Verification items for the finished model (mm, model axes). A direction names the side the tool comes from. Round coordinates to 2 decimals unless told otherwise and drop trailing zeros. Order: outer loops, then holes, each group sorted by start corner. A loop starts at its lowest first (then second) coordinate and runs counter-clockwise, first axis right, second up. Notation, with made-up numbers: (8, 62.5) -> (28, 62.5) arc R19 cw to (28, 82.5) -> close; hole circle Ø1 at (-19.75, 13.25). An arc over 180 degrees is marked (long way). Write item = value, one per line. Start each with the question number.
from build123d import *

# Parameters (mm, degrees)
BOSS_EXTRUDE1_DEPTH     = 18
SKETCH2_R               = 9.5
SKETCH2_W               = 9
SKETCH2_H               = 5.5
CUT_EXTRUDE1_DEPTH      = 51.410812332
FILLET1_R               = 5
FILLET2_R               = 0.5
FILLET3_R               = 2
FILLET4_R               = 2.75
CUT_EXTRUDE2_DEPTH      = 15
SKETCH7_R               = 1.6
CUT_EXTRUDE3_DEPTH      = 10
SKETCH8_R               = 2.35
CUT_EXTRUDE4_DEPTH      = 5
SKETCH9_R               = 2.5
CUT_EXTRUDE5_DEPTH      = 0.5
MIRROR3_COPY_1_SKETCH_R = 1.6
MIRROR3_COPY_1_DEPTH    = 10
MIRROR3_COPY_2_SKETCH_R = 2.35
MIRROR3_COPY_2_DEPTH    = 5
MIRROR3_COPY_3_SKETCH_R = 2.5
MIRROR3_COPY_3_DEPTH    = 0.5
BOSS_EXTRUDE2_DEPTH     = 27
SKETCH11_W              = 11
SKETCH11_H              = 20
CUT_EXTRUDE6_DEPTH      = 21.2
SKETCH12_W              = 11
SKETCH12_H              = 3.7
CUT_EXTRUDE7_DEPTH      = 12.5
FILLET5_R               = 10
CUT_EXTRUDE8_REACH      = 67.133
SKETCH13_W              = 11
SKETCH13_H              = 19.8
FILLET6_R               = 10
SKETCH14_W              = 11
SKETCH14_H              = 7.4
CUT_EXTRUDE9_DEPTH      = 12.5
SKETCH15_R              = 2.75
BOSS_EXTRUDE3_DEPTH     = 0.8
BOSS_EXTRUDE3_TAPER     = 30
SKETCH16_W              = 14
SKETCH16_H              = 6.815
CUT_EXTRUDE10_DEPTH     = 0.8
SKETCH19_R              = 2.75
BOSS_EXTRUDE4_DEPTH     = 0.8
BOSS_EXTRUDE4_TAPER     = 30
FILLET7_R               = 2


with BuildPart() as part:
    # Sketch1 → Boss-Extrude1 (new body)
    with BuildSketch(Plane.XY):
        with BuildLine():
            Line((-17.5, 17.5), (-31.5, 3.5))
            Line((-31.5, 3.5), (-31.5, -3.5))
            Line((-31.5, -3.5), (-17.5, -17.5))
            Line((-17.5, -17.5), (17.5, -17.5))
            Line((17.5, -17.5), (31.5, -3.5))
            Line((31.5, -3.5), (31.5, 3.5))
            Line((31.5, 3.5), (17.5, 17.5))
            Line((17.5, 17.5), (13.560660172, 17.5))
            Line((13.560660172, 17.5), (17.25, 13.810660172))
            Line((17.25, 13.810660172), (17.25, 9.845660172))
            Line((17.25, 9.845660172), (22.916347453, 4.179312718))
            ThreePointArc((22.916347453, 4.179312718), (22.602164744, -4.198757241), (21.880882362, 4.154117638))
            Line((21.880882362, 4.154117638), (16.5, 9.535))
            Line((16.5, 9.535), (16.5, 13.5))
            Line((16.5, 13.5), (12.5, 17.5))
            Line((12.5, 17.5), (-12.5, 17.5))
            Line((-12.5, 17.5), (-16.5, 13.5))
            Line((-16.5, 13.5), (-16.5, 9.535))
            Line((-16.5, 9.535), (-21.880882362, 4.154117638))
            ThreePointArc((-21.880882362, 4.154117638), (-22.602164744, -4.198757241), (-22.916347453, 4.179312718))
            Line((-22.916347453, 4.179312718), (-17.25, 9.845660172))
            Line((-17.25, 9.845660172), (-17.25, 13.810660172))
            Line((-17.25, 13.810660172), (-13.560660172, 17.5))
            Line((-13.560660172, 17.5), (-17.5, 17.5))
        make_face()
    extrude(amount=BOSS_EXTRUDE1_DEPTH)

    # Sketch2 → Cut-Extrude1 (cut, through all)
    with BuildSketch(Plane(origin=(0, 17.5, 0), x_dir=(1, 0, 0), z_dir=(0, 1, 0))):
        Circle(SKETCH2_R)
        with Locations((-5.5, -15.25)):
            Rectangle(SKETCH2_W, SKETCH2_H)
    extrude(amount=-CUT_EXTRUDE1_DEPTH, mode=Mode.SUBTRACT)

    # Fillet1
    fillet1_edges = [part.edges().sort_by_distance(p)[0] for p in [
        (17.5, 17.5, 9),
        (31.5, 3.5, 9),
        (31.5, -3.5, 9),
        (17.5, -17.5, 9),
        (-17.5, -17.5, 9),
        (-31.5, -3.5, 9),
        (-31.5, 3.5, 9),
        (-17.5, 17.5, 9),
    ]]
    fillet(fillet1_edges, radius=FILLET1_R)

    # Fillet2
    fillet2_edges = [part.edges().sort_by_distance(p)[0] for p in [
        (-13.560660172, 17.5, 9),
        (-22.916347453, 4.179312718, 9),
        (-21.880882362, 4.154117638, 9),
        (21.880882362, 4.154117638, 9),
        (22.916347453, 4.179312718, 9),
        (13.560660172, 17.5, 9),
    ]]
    fillet(fillet2_edges, radius=FILLET2_R)

    # Fillet3
    fillet3_edges = [part.edges().sort_by_distance(p)[0] for p in [
        (-17.25, 9.845660172, 9),
        (17.25, 9.845660172, 9),
    ]]
    fillet(fillet3_edges, radius=FILLET3_R)

    # Fillet4
    fillet4_edges = [part.edges().sort_by_distance(p)[0] for p in [
        (-16.5, 9.535, 9),
        (16.5, 9.535, 9),
    ]]
    fillet(fillet4_edges, radius=FILLET4_R)

    # Sketch4 → Cut-Revolve1 (revolve, cut)
    with BuildSketch(Plane(origin=(0, 0, 6), x_dir=(-1, 0, 0), z_dir=(0, 0, -1))):
        Polygon((23.439696962, 11.560303038), (25.561017306, 9.438982694), (23.439696962, 7.317662351), (22.555813485, 8.201545827), (14.070532111, -0.283735547), (12.833095244, 0.95370132), align=None)
    cut_revolve1 = revolve(axis=Axis((-23.439696962, 11.560303038, 6), (0.7071067811865471, -0.707106781186548, 0)), mode=Mode.SUBTRACT)

    # Sketch6 → Cut-Extrude2 (cut)
    with BuildSketch(Plane(origin=(-6.893398282, 6.893398282, 0), x_dir=(0, 0, 1), z_dir=(-0.7071067811865471, 0.707106781186548, 0))):
        Polygon((3.425, -9.886676943), (6, -11.373353886), (8.575, -9.886676943), (8.575, -6.913323057), (6, -5.426646114), (3.425, -6.913323057), align=None)
    cut_extrude2 = extrude(amount=-CUT_EXTRUDE2_DEPTH, mode=Mode.SUBTRACT)

    # Mirror1: Cut-Revolve1, Cut-Extrude2 across plane
    add(cut_revolve1.mirror(Plane(origin=(0, 0, 0), x_dir=(0, 0, 1), z_dir=(1, 0, 0))), mode=Mode.SUBTRACT)
    add(cut_extrude2.mirror(Plane(origin=(0, 0, 0), x_dir=(0, 0, 1), z_dir=(1, 0, 0))), mode=Mode.SUBTRACT)

    # Sketch7 → Cut-Extrude3 (cut)
    with BuildSketch(Plane(origin=(0, 0, 0), x_dir=(-1, 0, 0), z_dir=(0, 0, -1))):
        with Locations((-12.5, 12.5)):
            Circle(SKETCH7_R)
    cut_extrude3 = extrude(amount=-CUT_EXTRUDE3_DEPTH, mode=Mode.SUBTRACT)

    # Sketch8 → Cut-Extrude4 (cut)
    with BuildSketch(Plane(origin=(0, 0, 0), x_dir=(-1, 0, 0), z_dir=(0, 0, -1))):
        with Locations((-12.5, 12.5)):
            Circle(SKETCH8_R)
    cut_extrude4 = extrude(amount=-CUT_EXTRUDE4_DEPTH, mode=Mode.SUBTRACT)

    # Sketch9 → Cut-Extrude5 (cut)
    with BuildSketch(Plane(origin=(0, 0, 0), x_dir=(-1, 0, 0), z_dir=(0, 0, -1))):
        with Locations((-12.5, 12.5)):
            Circle(SKETCH9_R)
    cut_extrude5 = extrude(amount=-CUT_EXTRUDE5_DEPTH, mode=Mode.SUBTRACT)

    # Mirror2: Cut-Extrude3, Cut-Extrude4, Cut-Extrude5 across plane
    add(cut_extrude3.mirror(Plane.ZX), mode=Mode.SUBTRACT)
    add(cut_extrude4.mirror(Plane.ZX), mode=Mode.SUBTRACT)
    add(cut_extrude5.mirror(Plane.ZX), mode=Mode.SUBTRACT)

    # Mirror3: Cut-Extrude3, Cut-Extrude4, Cut-Extrude5 across plane
    add(cut_extrude3.mirror(Plane(origin=(0, 0, 0), x_dir=(0, 0, 1), z_dir=(1, 0, 0))), mode=Mode.SUBTRACT)
    add(cut_extrude4.mirror(Plane(origin=(0, 0, 0), x_dir=(0, 0, 1), z_dir=(1, 0, 0))), mode=Mode.SUBTRACT)
    add(cut_extrude5.mirror(Plane(origin=(0, 0, 0), x_dir=(0, 0, 1), z_dir=(1, 0, 0))), mode=Mode.SUBTRACT)

    # Mirror3 copy 1 sketch → Mirror3 copy 1 (cut)
    with BuildSketch(Plane(origin=(0, 0, 0), x_dir=(1, 0, 0), z_dir=(0, 0, -1))):
        with Locations((-12.5, 12.5)):
            Circle(MIRROR3_COPY_1_SKETCH_R)
    extrude(amount=-MIRROR3_COPY_1_DEPTH, mode=Mode.SUBTRACT)

    # Mirror3 copy 2 sketch → Mirror3 copy 2 (cut)
    with BuildSketch(Plane(origin=(0, 0, 0), x_dir=(1, 0, 0), z_dir=(0, 0, -1))):
        with Locations((-12.5, 12.5)):
            Circle(MIRROR3_COPY_2_SKETCH_R)
    extrude(amount=-MIRROR3_COPY_2_DEPTH, mode=Mode.SUBTRACT)

    # Mirror3 copy 3 sketch → Mirror3 copy 3 (cut)
    with BuildSketch(Plane(origin=(0, 0, 0), x_dir=(1, 0, 0), z_dir=(0, 0, -1))):
        with Locations((-12.5, 12.5)):
            Circle(MIRROR3_COPY_3_SKETCH_R)
    extrude(amount=-MIRROR3_COPY_3_DEPTH, mode=Mode.SUBTRACT)

    # Sketch10 → Boss-Extrude2 (add)
    with BuildSketch(Plane.XY.offset(18)):
        Polygon((12.5, 17.5), (-12.5, 17.5), (-16.5, 13.5), (-16.5, -13.5), (-12.5, -17.5), (12.5, -17.5), (16.5, -13.5), (16.5, 13.5), align=None)
    extrude(amount=BOSS_EXTRUDE2_DEPTH)

    # Sketch11 → Cut-Extrude6 (cut)
    with BuildSketch(Plane(origin=(0, 17.5, 0), x_dir=(1, 0, 0), z_dir=(0, 1, 0))):
        with Locations((5.5, -22.5)):
            Rectangle(SKETCH11_W, SKETCH11_H)
    extrude(amount=-CUT_EXTRUDE6_DEPTH, mode=Mode.SUBTRACT)

    # Sketch12 → Cut-Extrude7 (cut)
    with BuildSketch(Plane(origin=(0, 0, 32.5), x_dir=(-1, 0, 0), z_dir=(0, 0, -1))):
        with Locations((-5.5, 1.85)):
            Rectangle(SKETCH12_W, SKETCH12_H)
        Polygon((-11, -3.7), (0, -3.7), (0, -3.591245546), (0, 0), (-11, 0), align=None)
    extrude(amount=-CUT_EXTRUDE7_DEPTH, mode=Mode.SUBTRACT)

    # Fillet5
    fillet5_edges = [part.edges().sort_by_distance(p)[0] for p in [
        (5.5, -3.7, 12.5),
    ]]
    fillet(fillet5_edges, radius=FILLET5_R)

    # Cut-Extrude8: up to this face of the body (flat: up to its plane)
    cut_extrude8_end = Plane(part.part.faces().sort_by_distance((5.5, 3.7, 38.75))[0])
    # Sketch13 → Cut-Extrude8 (cut, up to the picked face)
    with BuildSketch(Plane.XZ.offset(17.5), mode=Mode.PRIVATE) as cut_extrude8_sk1:
        with Locations((-5.5, 35.1)):
            Rectangle(SKETCH13_W, SKETCH13_H)
    cut_extrude8_tool1 = split(extrude(cut_extrude8_sk1.sketch, amount=-CUT_EXTRUDE8_REACH, mode=Mode.PRIVATE), bisect_by=cut_extrude8_end, keep=Keep.BOTH, mode=Mode.PRIVATE)
    add(cut_extrude8_tool1.solids().sort_by(Axis((-5.5, -17.5, 35.1), (0, 1, 0)))[0], mode=Mode.SUBTRACT)

    # Fillet6
    # the kernel refuses this fillet: 10 mm, written as the material it adds along each edge
    with BuildSketch(Plane(origin=(25, 3.7, 25.2), x_dir=(0, 0, 1), z_dir=(-1, 0, 0))) as fillet6_piece_1_section:
        with BuildLine():
            CenterArc((FILLET6_R, -FILLET6_R), FILLET6_R, 90, 90)
            Line((0, -FILLET6_R), (0, 0))
            Line((0, 0), (FILLET6_R, 0))
        make_face()
    fillet6_piece_1 = extrude(amount=36, mode=Mode.PRIVATE)
    fillet6_piece_1 = split(fillet6_piece_1, bisect_by=Plane(origin=(5.5, 3.588944861, 32.5), z_dir=(0, 0, 1)), keep=Keep.TOP, mode=Mode.PRIVATE)
    fillet6_piece_1 = split(fillet6_piece_1, bisect_by=Plane(origin=(11, 3.588944861, 33.172467691), z_dir=(-1, 0, 0)), keep=Keep.TOP, mode=Mode.PRIVATE)
    add(fillet6_piece_1)
    with BuildSketch(Plane(origin=(0, 3.7, 25.2), x_dir=(0, 0, 1), z_dir=(-1, 0, 0))) as fillet6_piece_2:
        with BuildLine():
            CenterArc((FILLET6_R, -FILLET6_R), FILLET6_R, 90, 90)
            Line((0, -FILLET6_R), (0, 0))
            Line((0, 0), (FILLET6_R, 0))
        make_face()
    extrude(amount=11)

    # Sketch14 → Cut-Extrude9 (cut)
    with BuildSketch(Plane.XY.offset(45)):
        with Locations((5.5, 0)):
            Rectangle(SKETCH14_W, SKETCH14_H)
    extrude(amount=-CUT_EXTRUDE9_DEPTH, mode=Mode.SUBTRACT)

    # Sketch15 → Boss-Extrude3 (add)
    with BuildSketch(Plane(origin=(-11, 0, 0), x_dir=(0, 0, -1), z_dir=(1, 0, 0))):
        with Locations((-35.23, -6.365)):
            Circle(SKETCH15_R)
    extrude(amount=BOSS_EXTRUDE3_DEPTH, taper=BOSS_EXTRUDE3_TAPER)

    # Sketch16 → Cut-Extrude10 (cut)
    with BuildSketch(Plane.ZY):
        with Locations((38, -7.1075)):
            Rectangle(SKETCH16_W, SKETCH16_H)
    extrude(amount=-CUT_EXTRUDE10_DEPTH, mode=Mode.SUBTRACT)

    # Sketch17 → Cut-Revolve2 (revolve, cut)
    with BuildSketch(Plane.XY.offset(35.23)):
        Polygon((-16.5, -6.365), (-16.5, -3.265), (-13.5, -3.265), (-13.5, -4.865), (11.5, -4.865), (11.5, -4.115), (16, -4.115), (16, -3.865), (16.5, -3.865), (16.5, -6.365), align=None)
    revolve(axis=Axis((31.947720378, -6.365, 35.23), (-1, 0, 0)), mode=Mode.SUBTRACT)

    # Sketch19 → Boss-Extrude4 (add)
    with BuildSketch(Plane.ZY.offset(-11)):
        with Locations((22.5, 6.365)):
            Circle(SKETCH19_R)
    boss_extrude4 = extrude(amount=BOSS_EXTRUDE4_DEPTH, taper=BOSS_EXTRUDE4_TAPER)

    # Mirror4: Boss-Extrude4 across plane
    add(boss_extrude4.mirror(Plane(origin=(5.5, 0, 0), x_dir=(0, 0, 1), z_dir=(1, 0, 0))))

    # Sketch20 → Cut-Revolve3 (revolve, cut)
    with BuildSketch(Plane.XY.offset(22.5), mode=Mode.PRIVATE) as cut_revolve3_sk:
        Polygon((16.5, 6.365), (16.5, 9.465), (13.5, 9.465), (13.5, 7.865), (-11.5, 7.865), (-11.5, 8.615), (-16, 8.615), (-16, 8.865), (-16.5, 8.865), (-16.5, 6.365), align=None)
    revolve(cut_revolve3_sk.sketch.rotate(Axis((11, 6.365, 22.5), (-1, 0, 0)), 90), axis=Axis((11, 6.365, 22.5), (-1, 0, 0)), mode=Mode.SUBTRACT)

    # Fillet7
    fillet7_edges = [part.edges().sort_by_distance(p)[0] for p in [
        (16.5, -13.5, 31.5),
        (12.5, -17.5, 31.5),
        (-12.5, -17.5, 31.5),
        (-16.5, -13.5, 31.5),
        (-16.5, 13.5, 22.5),
        (-12.5, 17.5, 22.5),
        (12.5, 17.5, 22.5),
        (16.5, 13.5, 22.5),
    ]]
    fillet(fillet7_edges, radius=FILLET7_R)


solid = part.part
(1) Scan lines: line 1 along X through (y, z) = (-12.5, 3.15); line 2 along X through (y, z) = (-1, 42); line 3 along X through (y, z) = (6, 19.5). Record each from-to range of solid material in increasing order. Write a range as from..to.
(2) Draft check along Y on faces 6 (the flat face through (5, 12, 12.5)), 7 (the cylindrical face through (16.35, -13.43, 31.69)), 8 (the flat face through (-11, -1, 3.425)), 9 (the cylindrical face through (-22.77, -4.19, 8.87)). Enter one of: +Y half, -Y half, draft (parallel to the pull), parting line (faces both ways), or undercut.
(3) Depth check by flat-ended pin: pin 1 (2.5 mm diameter, centred on y = 6.365, z = 22.5, fed in from -X); pin 2 (6.5 mm diameter, centred on y = -6.365, z = 35.23, fed in from +X); pin 3 (4 mm diameter, centred on x = 15.5, z = 38.5, fed in from +Y); pin 4 (2.5 mm diameter, centred on x = -4.5, y = 7.5, fed in from -Z). Enter the tip coordinate at first touch or a pass-through.
(4) Set-up check for faces 1 (the cylindrical face through (-5.4, 6.3, 24)), 2 (the cylindrical face through (14.1, -12.57, 7.46)), 3 (the flat face through (-9.59, 0.88, 4.73)), 4 (the flat face through (-11.5, 8, 23)), 5 (the cylindrical face through (16.715, 9.608, 9.126)): record each of +Z, -Z, +X, -X, +Y, -Y from which the full face is reachable in a straight line by a thin tool's end or side.
(5) Cross-section at A-A (z = 40.5). Enter the section's corners in (x, y) (3 decimals), and give its area (3 significant figures).
Outcome:
q1.line_1 = -22.5..-14.85, -10.15..-8.96, 8.96..10.15, 14.85..22.5
q1.line_2 = -16.5..-11, 11..16.5
q1.line_3 = -16.5..0, 11..13.5
q2.face_6 = draft
q2.face_7 = -Y half
q2.face_8 = undercut
q2.face_9 = undercut
q3.pin_1 = through
q3.pin_2 = 16.5
q3.pin_3 = 16.5
q3.pin_4 = 7.56
q4.face_1 = +X, -X
q4.face_2 = -Z
q4.face_3 = none
q4.face_4 = -X
q4.face_5 = +Z, -Z
q5.outline = (-16.5, -12.672) arc R2 ccw to (-15.914, -14.086) -> (-13.086, -16.914) arc R2 ccw to (-11.672, -17.5) -> (-11, -17.5) -> (-11, 3.7) -> (11, 3.7) -> (11, -3.7) -> (0.8, -3.7) -> (0.8, -10.515) -> (0, -10.515) -> (0, -17.5) -> (11.672, -17.5) arc R2 ccw to (13.086, -16.914) -> (15.914, -14.086) arc R2 ccw to (16.5, -12.672) -> (16.5, 12.672) arc R2 ccw to (15.914, 14.086) -> (13.086, 16.914) arc R2 ccw to (11.672, 17.5) -> (-11.672, 17.5) arc R2 ccw to (-13.086, 16.914) -> (-15.914, 14.086) arc R2 ccw to (-16.5, 12.672) -> close
q5.area = 802 mm^2
